from build123d import *

# Parameters (mm, degrees)
SKETCH3_R                                    = 1.5
BOSS_EXTRUDE2_DEPTH                          = 40
SKETCH4_W                                    = 6
SKETCH4_H                                    = 20
CUT_EXTRUDE1_DEPTH                           = 40
CUT_EXTRUDE1_DEPTH_BACK                      = 200
FILLET1_R                                    = 1
FILLET2_R                                    = 1
CSK_FOR_M2_5_COUNTERSUNK_FLAT_HEAD_S_2_COUNT = 2
CSK_FOR_M2_5_COUNTERSUNK_FLAT_HEAD_S_2_PITCH = 15
CSK_FOR_M2_5_COUNTERSUNK_FLAT_HEAD_S_3_COUNT = 2
CSK_FOR_M2_5_COUNTERSUNK_FLAT_HEAD_S_3_PITCH = 30


with BuildPart() as part:
    # Sketch3 → Boss-Extrude2 (new body)
    with BuildSketch(Plane(origin=(0, 0, 0), x_dir=(1, 0, 0), z_dir=(0, 1, 0))):
        with BuildLine():
            Line((-5, 1), (5, 1))
            Line((5, 1), (5, -1))
            Line((5, -1), (-5, -1))
            ThreePointArc((-5, -1), (-7.043086083, 0.276738431), (-9.332231573, 1.027787491))
            ThreePointArc((-9.332231573, 1.027787491), (-10.291421088, 4.527164553), (-7, 3))
            ThreePointArc((-7, 3), (-6.182675814, 1.817324186), (-5, 1))
        make_face()
        with Locations((-9, 3)):
            Circle(SKETCH3_R, mode=Mode.SUBTRACT)
    extrude(amount=BOSS_EXTRUDE2_DEPTH)

    # Sketch4 → Cut-Extrude1 (cut, two sides)
    with BuildSketch(Plane.XY) as cut_extrude1_sk:
        with Locations((-8, 20)):
            Rectangle(SKETCH4_W, SKETCH4_H)
    extrude(amount=CUT_EXTRUDE1_DEPTH, mode=Mode.SUBTRACT)
    extrude(cut_extrude1_sk.sketch, amount=-CUT_EXTRUDE1_DEPTH_BACK, mode=Mode.SUBTRACT)

    # Fillet1
    fillet1_edges = [part.edges().sort_by_distance(p)[0] for p in [
        (5, 20, -1),
        (-5, 20, -1),
    ]]
    fillet(fillet1_edges, radius=FILLET1_R)

    # Fillet2
    fillet2_edges = [part.edges().sort_by_distance(p)[0] for p in [
        (-6.182675814, 40, -1.817324186),
        (-5, 35, -1),
        (-5, 5, -1),
        (5, 40, 0.5),
        (-0.5, 0, -1),
        (-0.5, 40, -1),
        (4.707106781, 0, -0.707106781),
        (4.707106781, 40, -0.707106781),
        (-6.182675814, 0, -1.817324186),
        (5, 0, 0.5),
    ]]
    fillet(fillet2_edges, radius=FILLET2_R)

    # Sketch6 → CSK for M2.5 Countersunk Flat Head Screw1 (revolve, cut)
    with BuildSketch(Plane(origin=(0, 35, -1), x_dir=(0, 1, 0), z_dir=(1, 0, 0))):
        Polygon((0, 0), (0, 2), (1.45, 2), (1.45, 1.3), (2.75, 0), align=None)
    csk_for_m2_5_countersunk_flat_head_screw = revolve(axis=Axis((0, 35, -7.35), (0, 0, 1)), mode=Mode.SUBTRACT)

    # CSK for M2.5 Countersunk Flat Head S 2: CSK for M2.5 Countersunk Flat Head Screw1 ×2
    with Locations(*[(0, -i * CSK_FOR_M2_5_COUNTERSUNK_FLAT_HEAD_S_2_PITCH, 0) for i in range(1, CSK_FOR_M2_5_COUNTERSUNK_FLAT_HEAD_S_2_COUNT)]):
        add(csk_for_m2_5_countersunk_flat_head_screw, mode=Mode.SUBTRACT)

    # CSK for M2.5 Countersunk Flat Head S 3: CSK for M2.5 Countersunk Flat Head Screw1 ×2
    with Locations(*[(0, -i * CSK_FOR_M2_5_COUNTERSUNK_FLAT_HEAD_S_3_PITCH, 0) for i in range(1, CSK_FOR_M2_5_COUNTERSUNK_FLAT_HEAD_S_3_COUNT)]):
        add(csk_for_m2_5_countersunk_flat_head_screw, mode=Mode.SUBTRACT)


solid = part.part
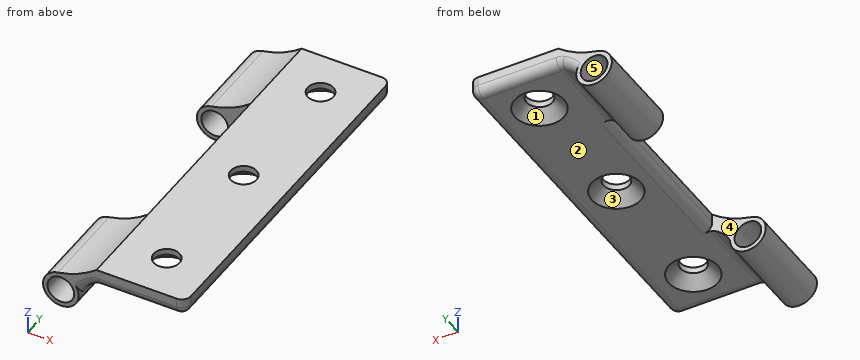
Geometry: final body of the model. Coordinates: model frame, mm. Face numbers are marked on the shaded views. A direction names the side the tool comes from. Round coordinates to 2 decimals unless told otherwise and drop trailing zeros. Order: outer loops, then holes, each group sorted by start corner. A loop starts at its lowest first (then second) coordinate and runs counter-clockwise, first axis right, second up.
Q1. Section A-A, the plane y = 35. Output: boundary loops of the cut face in (x, z).
Result sheet:
outline: (-9.33, -1.03) arc R2 ccw (long way) to (-7, -3) arc R4 cw to (-5.24, -1.12) arc R1 cw to (-4.77, -1) - (-2.75, -1) - (-1.45, 0.3) - (-1.45, 1) - (-5, 1) arc R10 cw to start; (1.45, 0.3) - (2.75, -1) - (4, -1) arc R1 ccw to (5, 0) - (5, 1) - (1.45, 1) - close; hole circle Ø3 at (-9, -3)
Q2. Section B-B, the plane x = 0. Output: boundary loops of the cut face in (y, z), and give its area (3 significant figures).
Result sheet:
outline: (0, 0) arc R1 ccw to (1, -1) - (2.25, -1) - (3.55, 0.3) - (3.55, 1) - (0, 1) - close; (6.45, 0.3) - (7.75, -1) - (17.25, -1) - (18.55, 0.3) - (18.55, 1) - (6.45, 1) - close; (21.45, 0.3) - (22.75, -1) - (32.25, -1) - (33.55, 0.3) - (33.55, 1) - (21.45, 1) - close; (36.45, 0.3) - (37.75, -1) - (39, -1) arc R1 ccw to (40, 0) - (40, 1) - (36.45, 1) - close
area: 57.1 mm2
Q3. Mould query, pull axis Z, two halves, no side actions, for the marked faces 3, 4 and 5. Classes: released by +Z, released by -Z, zero draft, split by the parting line, or undercut.
Result sheet:
face 3: released by -Z
face 4: zero draft
face 5: undercut
Q4. Access query for the marked faces 1 and 2. Directions: +Z, -Z, +X, -X, +Y, -Y. A direction counts if a zero-diameter tool reaches every point of the face in a straight line with its end or side. Return the directions, or none.
Result sheet:
face 1: -Z
face 2: -Z, +X, +Y, -Y
Q5. Material intervals for probe 1 along Y at (x, z) = (-0.5, 0.5); probe 2 along X at (y, z) = (35.25, -3); probe 3 along X at (y, z) = (20, 0.85), sorted ascending.
Result sheet:
probe 1: y = 0 to 3.64, 6.36 to 18.64, 21.36 to 33.64, 36.36 to 40
probe 2: x = -11 to -10.5, -7.5 to -7
probe 3: x = -5 to -1.45, 1.45 to 5
Q6. Section D-D, the plane z = -3.75. Output: boundary loops of the cut face in (x, y).
Result sheet:
outline: (-10.85, 0) - (-10.3, 0) - (-10.3, 10) - (-10.85, 10) - close; (-10.85, 30) - (-10.3, 30) - (-10.3, 40) - (-10.85, 40) - close; (-7.7, 0) - (-7.15, 0) - (-7.15, 10) - (-7.7, 10) - close; (-7.7, 30) - (-7.15, 30) - (-7.15, 40) - (-7.7, 40) - close
Q7. Pin query (flat end, axial travel): pin 1 (1 mm diameter, centred on y = 5, z = -2, fed in from -X); pin 2 (0.5 mm diameter, centred on y = 23, z = 0.5, fed in from -X); pin 3 (4 mm diameter, centred on x = 0, y = 20, fed in from -Z). Return the tip coordinate at first contact, or that it passes through.
Result sheet:
pin 1: stops at x = -10.94
pin 2: stops at x = -5
pin 3: stops at z = -0.25
Q8. Section C-C, the plane y = 9. Output: boundary loops of the cut face in (x, z), and give its area (3 significant figures).
Result sheet:
outline: (-9.33, -1.03) arc R2 ccw (long way) to (-7, -3) arc R4 cw to (-5.24, -1.12) arc R1 cw to (-4.77, -1) - (4, -1) arc R1 ccw to (5, 0) - (5, 1) - (-5, 1) arc R10 cw to start; hole circle Ø3 at (-9, -3)
area: 31.0 mm2
